Input: part model. Units: mm. Frame: model coordinates. Round coordinates to 2 decimals unless told otherwise and drop trailing zeros. Loops run counter-clockwise (first coordinate to the right, second up) from the corner with the lowest first, then second, coordinate; pieces in that order, holes last. Notation, with made-up numbers: M 12.25,32.5 L 19.25,32.5 A18 cw 19.25,39.5 Z; hole C 73,-9 d11. An arc over 180 degrees is marked long. Use one line per item in the form item = value. Start each with the question number.
Q1. Mould query, pull axis Z, two halves, no side actions, for faces 1 (the flat face through (-213.42, 95.89, 3.85)), 2 (the flat face through (-212.249, 98.846, 5.944)), 3 (the flat face through (-214.7, 93.3, 0.5)), 4 (the flat face through (-210.67, 101.52, 7.97)). Classes: pulls with the +Z half, pulls with the -Z half, needs draft (parallel to the pull), parting line crosses it, or undercut.
Q2. Ray query, line 1 along Y through (x, z) = (-213.75, 10); line 2 along X through (y, z) = (93.5, 8.75); line 3 along Y through (x, z) = (-209.25, 6.25). Return the intervals inside material, ascending.
Q3. Section query C-C, the plane x = -213.5. Output: boundary loops of the cut face in (y, z), and give its area (3 significant figures).
Q4. First-contact query: P1, Ø1.5, axis at y = 96.5, z = 1.5, coming from the -X side; P2, Ø1, axis at x = -214, z = 10, coming from the +Y side; P3, Ø0.5, axis at x = -209, y = 104.5, coming from the +Z side; P4, Ø3, axis at x = -213, y = 95.5, coming from the -Z side. Flat tips, straight axial feed; report the tip coordinate or a pass-through.
Q5. Section query B-B, the plane z = 8. Output: boundary loops of the cut face in (x, y), and give its area (3 significant figures).
Q6. Section query A-A, the plane y = 99.75. Output: boundary loops of the cut face in (x, z).
```python
from build123d import *

# Parameters (mm, degrees)
BOX212_W                  = 0.5
BOX212_H                  = 1
BOX212_DEPTH              = 11
BOX213_W                  = 0.5
BOX213_H                  = 1
BOX213_DEPTH              = 16
BOX213_ROLL_ANGLE         = 49
BOX214_W                  = 0.5
BOX214_H                  = 1
BOX214_DEPTH              = 16
BOX214_ROLL_ANGLE         = -49
BOX211_W                  = 0.5
BOX211_H                  = 1
BOX211_DEPTH              = 11
FUSION015_PLACEMENT_ANGLE = -26


with BuildPart() as cubo212:
    # Box212 → Box212 (new body)
    with BuildSketch(Plane(origin=(0, 12, 0.5), x_dir=(1, 0, 0), z_dir=(0, 0, 1))):
        with Locations((0.25, 0.5)):
            Rectangle(BOX212_W, BOX212_H)
    extrude(amount=BOX212_DEPTH)


with BuildPart() as cubo213:
    # Box213 → Box213 (new body)
    with BuildSketch(Plane.XY):
        with Locations((0.25, 0.5)):
            Rectangle(BOX213_W, BOX213_H)
    extrude(amount=BOX213_DEPTH)


with BuildPart() as cubo213_1:
    # Box213 roll: moved
    add(cubo213.part.rotate(Axis((0, 0, 0), (1, 0, 0)), BOX213_ROLL_ANGLE))


with BuildPart() as cubo213_2:
    # Box213 placement: moved
    add(cubo213_1.part.moved(Location((0, 12, 0.5))))


with BuildPart() as cubo214:
    # Box214 → Box214 (new body)
    with BuildSketch(Plane.XY):
        with Locations((0.25, 0.5)):
            Rectangle(BOX214_W, BOX214_H)
    extrude(amount=BOX214_DEPTH)


with BuildPart() as cubo214_1:
    # Box214 roll: moved
    add(cubo214.part.rotate(Axis((0, 0, 0), (1, 0, 0)), BOX214_ROLL_ANGLE))


with BuildPart() as cubo214_2:
    # Box214 placement: moved
    add(cubo214_1.part.moved(Location((0, 0.4, 1.3))))


with BuildPart() as fusion015:
    # Box211 → Box211 (new body)
    with BuildSketch(Plane.XY.offset(0.5)):
        with Locations((0.25, 0.5)):
            Rectangle(BOX211_W, BOX211_H)
    extrude(amount=BOX211_DEPTH)

    # Fusion015: union Cubo212, Cubo213, Cubo214
    add(cubo212.part)
    add(cubo213_2.part)
    add(cubo214_2.part)


with BuildPart() as fusion015_1:
    # Fusion015 placement: moved
    add(fusion015.part.moved(Location((-215.1, 93, 0))).rotate(Axis((-215.1, 93, 0), (0, 0, 1)), FUSION015_PLACEMENT_ANGLE))


solid = fusion015_1.part
```
Results found:
q1.face_1 = undercut
q1.face_2 = needs draft
q1.face_3 = pulls with the -Z half
q1.face_4 = undercut
q2.line_1 = 94.63 to 95.23
q2.line_2 = -214.86 to -214.3
q2.line_3 = 103.85 to 104.61
q3.outline = M 95.14,1.91 L 96.28,2.8 L 96.28,4.13 L 95.14,3.23 Z; M 95.14,8.65 L 96.28,7.76 L 96.28,9.08 L 95.14,9.97 Z
q3.area = 3.02 mm²
q4.P1 = through
q4.P2 = 95.78
q4.P3 = 11.5
q4.P4 = 1.1
q5.outline = M -215.1,93 L -214.65,92.78 L -214.21,93.68 L -214.66,93.9 Z; M -213.62,96.03 L -213.17,95.81 L -212.5,97.18 L -212.95,97.4 Z; M -211.55,100.29 L -211.1,100.07 L -210.43,101.44 L -210.88,101.66 Z; M -209.84,103.79 L -209.39,103.57 L -208.95,104.47 L -209.4,104.68 Z
q5.area = 2.52 mm²
q6.outline = M -211.81,4.4 L -211.25,4.19 L -211.25,5.52 L -211.81,5.73 Z; M -211.81,6.16 L -211.25,6.37 L -211.25,7.69 L -211.81,7.48 Z
